from build123d import *

# Parameters (mm, degrees)
SKETCH1_R           = 1.85
SKETCH1_R_2         = 1.5
SKETCH1_R_3         = 1.65
SKETCH1_R_4         = 43
BOSS_EXTRUDE1_DEPTH = 5.842
FILLET1_R           = 4
BOSS_EXTRUDE2_DEPTH = 5.842
FILLET2_R           = 3


with BuildPart() as part:
    # Sketch1 → Boss-Extrude1 (new body)
    # profile 1 of 2: a face of its own
    with BuildSketch(Plane.XY):
        with BuildLine():
            ThreePointArc((50.8, 0), (0, 50.8), (-50.8, 0))
            Line((-50.8, 0), (-50.8, -57.658))
            Line((-50.8, -57.658), (0, -57.658))
            Line((0, -57.658), (50.8, -57.658))
            Line((50.8, -57.658), (50.8, 0))
        make_face()
        with Locations((-41.8, -47.658)):
            Circle(SKETCH1_R, mode=Mode.SUBTRACT)
        with Locations((-33.855565576, -33.855565576)):
            Circle(SKETCH1_R_2, mode=Mode.SUBTRACT)
        with Locations((-41.8, -27.658)):
            Circle(SKETCH1_R, mode=Mode.SUBTRACT)
        with Locations((0, -47.879)):
            Circle(SKETCH1_R_3, mode=Mode.SUBTRACT)
        with Locations((41.8, -47.658)):
            Circle(SKETCH1_R, mode=Mode.SUBTRACT)
        with Locations((33.855565576, -33.855565576)):
            Circle(SKETCH1_R_2, mode=Mode.SUBTRACT)
        with Locations((41.8, -27.658)):
            Circle(SKETCH1_R, mode=Mode.SUBTRACT)
        with Locations((-47.879, 0)):
            Circle(SKETCH1_R_3, mode=Mode.SUBTRACT)
        Circle(SKETCH1_R_4, mode=Mode.SUBTRACT)
        with Locations((-33.855565576, 33.855565576)):
            Circle(SKETCH1_R_2, mode=Mode.SUBTRACT)
        with Locations((0, 47.879)):
            Circle(SKETCH1_R_3, mode=Mode.SUBTRACT)
        with Locations((47.879, 0)):
            Circle(SKETCH1_R_3, mode=Mode.SUBTRACT)
        with Locations((33.855565576, 33.855565576)):
            Circle(SKETCH1_R_2, mode=Mode.SUBTRACT)
    # profile 2 of 2: a face of its own
    with BuildSketch(Plane.XY):
        with BuildLine():
            ThreePointArc((50.8, 0), (0, 50.8), (-50.8, 0))
            Line((-50.8, 0), (-50.8, -57.658))
            Line((-50.8, -57.658), (0, -57.658))
            Line((0, -57.658), (50.8, -57.658))
            Line((50.8, -57.658), (50.8, 0))
        make_face()
        with Locations((-41.8, -47.658)):
            Circle(SKETCH1_R, mode=Mode.SUBTRACT)
        with Locations((-33.855565576, -33.855565576)):
            Circle(SKETCH1_R_2, mode=Mode.SUBTRACT)
        with Locations((-41.8, -27.658)):
            Circle(SKETCH1_R, mode=Mode.SUBTRACT)
        with Locations((0, -47.879)):
            Circle(SKETCH1_R_3, mode=Mode.SUBTRACT)
        with Locations((41.8, -47.658)):
            Circle(SKETCH1_R, mode=Mode.SUBTRACT)
        with Locations((33.855565576, -33.855565576)):
            Circle(SKETCH1_R_2, mode=Mode.SUBTRACT)
        with Locations((41.8, -27.658)):
            Circle(SKETCH1_R, mode=Mode.SUBTRACT)
        with Locations((-47.879, 0)):
            Circle(SKETCH1_R_3, mode=Mode.SUBTRACT)
        Circle(SKETCH1_R_4, mode=Mode.SUBTRACT)
        with Locations((-33.855565576, 33.855565576)):
            Circle(SKETCH1_R_2, mode=Mode.SUBTRACT)
        with Locations((0, 47.879)):
            Circle(SKETCH1_R_3, mode=Mode.SUBTRACT)
        with Locations((47.879, 0)):
            Circle(SKETCH1_R_3, mode=Mode.SUBTRACT)
        with Locations((33.855565576, 33.855565576)):
            Circle(SKETCH1_R_2, mode=Mode.SUBTRACT)
    extrude(amount=BOSS_EXTRUDE1_DEPTH)

    # Fillet1
    fillet1_edges = [part.edges().sort_by_distance(p)[0] for p in [
        (50.8, -57.658, 2.921),
        (-50.8, -57.658, 2.921),
    ]]
    fillet(fillet1_edges, radius=FILLET1_R)

    # Sketch2 → Boss-Extrude2 (add, through all)
    with BuildSketch(Plane.XY.offset(5.842)):
        Polygon((-50.592347052, 4.588509541), (-90.8, 4.588509541), (-90.8, -39.411490459), (-50.8, -39.411490459), align=None)
        with BuildLine():
            Line((-67.8, -33.411490459), (-72.8, -33.411490459))
            ThreePointArc((-72.8, -33.411490459), (-88.8, -17.411490459), (-72.8, -1.411490459))
            Line((-72.8, -1.411490459), (-67.8, -1.411490459))
            ThreePointArc((-67.8, -1.411490459), (-51.8, -17.411490459), (-67.8, -33.411490459))
        make_face(mode=Mode.SUBTRACT)
        with BuildLine():
            Line((-79.8, -1.061490459), (-84.8, -1.061490459))
            ThreePointArc((-84.8, -1.061490459), (-86.45, 0.588509541), (-84.8, 2.238509541))
            Line((-84.8, 2.238509541), (-79.8, 2.238509541))
            ThreePointArc((-79.8, 2.238509541), (-78.15, 0.588509541), (-79.8, -1.061490459))
        make_face(mode=Mode.SUBTRACT)
        with BuildLine():
            Line((-55.8, -1.061490459), (-60.8, -1.061490459))
            ThreePointArc((-60.8, -1.061490459), (-62.45, 0.588509541), (-60.8, 2.238509541))
            Line((-60.8, 2.238509541), (-55.8, 2.238509541))
            ThreePointArc((-55.8, 2.238509541), (-54.15, 0.588509541), (-55.8, -1.061490459))
        make_face(mode=Mode.SUBTRACT)
        with BuildLine():
            Line((-55.8, -37.061490459), (-60.8, -37.061490459))
            ThreePointArc((-60.8, -37.061490459), (-62.45, -35.411490459), (-60.8, -33.761490459))
            Line((-60.8, -33.761490459), (-55.8, -33.761490459))
            ThreePointArc((-55.8, -33.761490459), (-54.15, -35.411490459), (-55.8, -37.061490459))
        make_face(mode=Mode.SUBTRACT)
        with BuildLine():
            Line((-79.8, -37.061490459), (-84.8, -37.061490459))
            ThreePointArc((-84.8, -37.061490459), (-86.45, -35.411490459), (-84.8, -33.761490459))
            Line((-84.8, -33.761490459), (-79.8, -33.761490459))
            ThreePointArc((-79.8, -33.761490459), (-78.15, -35.411490459), (-79.8, -37.061490459))
        make_face(mode=Mode.SUBTRACT)
    extrude(amount=-BOSS_EXTRUDE2_DEPTH)

    # Fillet2
    fillet2_edges = [part.edges().sort_by_distance(p)[0] for p in [
        (-50.592347052, 4.588509541, 2.921),
        (-50.8, -39.411490459, 2.921),
        (-90.8, -39.411490459, 2.921),
        (-90.8, 4.588509541, 2.921),
    ]]
    fillet(fillet2_edges, radius=FILLET2_R)


solid = part.part
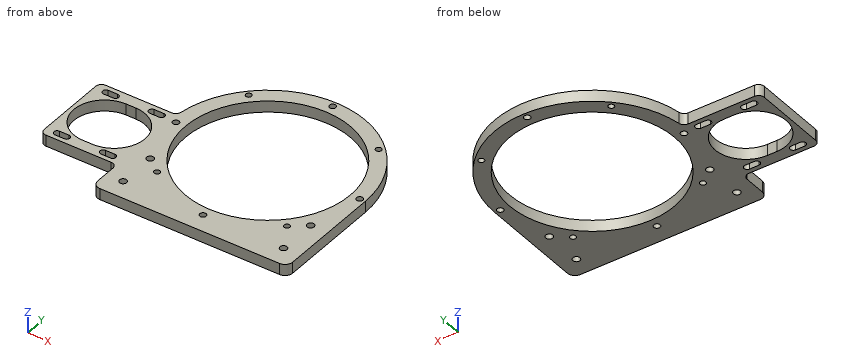
The listing builds one solid part. Answer for the finished solid, in the listing's coordinates (mm). Coordinates: 2 decimals unless noted, no trailing zeros. Loops run counter-clockwise (first coordinate to the right, second up) from the corner with the lowest first, then second, coordinate; pieces in that order, holes last. Notation, with made-up numbers: M 65,79.5 L 88,79.5 A18 ccw 88,104.5 Z; hole C 31.25,48.5 d10. An arc over 180 degrees is marked long. Answer in a Markdown table with one row per item.
1) Given pin 1 (3 mm diameter, centred on x = 24, z = 3.5, fed in from +Y); pin 2 (1.8 mm diameter, centred on x = -63.5, z = 3.5, fed in from -Y); pin 3 (1 mm diameter, centred on x = -54, z = 5, fed in from +Y), each flat-ended and moving along its own axis, determine where each tip first touches the part or whether it passes through.
Answers below:
| item | result |
|---|---|
| pin 1 | y = 45.55 |
| pin 2 | y = -39.41 |
| pin 3 | y = 4.59 |
2) Find the intervals of material crossed by probe 1 along Y at (x, z) = (-70.5, 5.3); probe 2 along X at (y, z) = (-35, 1.6); probe 3 along X at (y, z) = (-48.5, 3.75), in increasing order.
Answers below:
| item | result |
|---|---|
| probe 1 | -39.41 to -33.41, -1.41 to 4.59 |
| probe 2 | -90.8 to -86.4, -78.2 to -62.4, -54.2 to -34.83, -32.89 to -24.98, 24.98 to 32.89, 34.83 to 50.8 |
| probe 3 | -50.8 to -43.45, -40.15 to -1.53, 1.53 to 40.15, 43.45 to 50.8 |
3) Find section B-B (y = -9). Determine the outline of the cut face in (x, z), then the cut area to 3 significant figures.
Answers below:
| item | result |
|---|---|
| outline | M -90.8,0 L -86.41,0 L -86.41,5.84 L -90.8,5.84 Z; M -54.19,0 L -42.05,0 L -42.05,5.84 L -54.19,5.84 Z; M 42.05,0 L 50.8,0 L 50.8,5.84 L 42.05,5.84 Z |
| area | 148 mm^2 |
4) Find section A-A (x = 0). Determine the outline of the cut face in (y, z).
Answers below:
| item | result |
|---|---|
| outline | M -57.66,0 L -49.53,0 L -49.53,5.84 L -57.66,5.84 Z; M -46.23,0 L -43,0 L -43,5.84 L -46.23,5.84 Z; M 43,0 L 46.23,0 L 46.23,5.84 L 43,5.84 Z; M 49.53,0 L 50.8,0 L 50.8,5.84 L 49.53,5.84 Z |
